Build history of the part. All positions in model axes, mm. A direction names the side the tool comes from. Give positions to 0.01 mm unless a question says otherwise; leave off trailing zeros. Loops run counter-clockwise (first coordinate to the right, second up) from the corner with the lowest first, then second, coordinate; pieces in that order, holes last. Notation, with made-up numbers: (41.25, -19) - (61.25, -19) arc R32 cw to (61.25, 13) - close; hole circle Ø5 at (21.25, 18). An arc over 180 degrees is marked (long way). Return JSON: item names as keys, results as strings. Group by question number.
1) Drill centre lines: probe 1 along X at (y, z) = (8, 28); probe 2 along Y at (x, z) = (-30.5, 8); probe 3 along Z at (x, y) = (-29, 7.75). Where is each one in solid material? Low to high. Write a range as from..to.
2) Slice it at B-B (z = 11). List the corners of the cut face in (x, y), and give its area (3 significant figures).
3) 3-axis set-ups, long thin cutter, end or side, ignore diameter. For faces 5 (the face through (-35, 15, 67)), 6 (the face through (0, 14, 35)): which of +Z, -Z, +X, -X, +Y, -Y reach the whole face in a straight line?
4) Drop flat-ended pins along their axis: pin 1 (8 mm diameter, centred on x = -42.5, y = 22, fed in from -Z); pin 2 (1.5 mm diameter, centred on x = -14.5, z = 21, fed in from -Y); pin 3 (6 mm diameter, centred on x = -13, z = 24.5, fed in from +Y); pin 4 (5 mm diameter, centred on x = -59, y = 21.5, fed in from -Z). Give the stop position or say it passes through.
5) Mould opens along Z. For faces 1 (the face through (-35, 0, 35)), 2 (the face through (-67, 15, 44)), 3 (the face through (-36.732, 14.11, 0.813)), 4 (the face through (-41.052, 14.035, -2.396)) say: released by +Z, released by -Z, zero draft, split by the parting line, or undercut.
6) Slice it at C-C (x = -24). List the corners of the cut face in (y, z).
7) Slice it at A-A (y = 5.75). List the corners of the cut face in (x, z).
```python
from build123d import *

# Parameters (mm, degrees)
BOSS_EXTRUDE1_DEPTH             = 3
BOSS_EXTRUDE2_DEPTH             = 25
SKETCH4_R                       = 2.5
BOSS_EXTRUDE3_DEPTH             = 7
BOSS_EXTRUDE3_DIRECTION_2_REACH = 85.256


with BuildPart() as part:
    # Sketch1 → Boss-Extrude1 (new body)
    with BuildSketch(Plane(origin=(0, 0, 0), x_dir=(1, 0, 0), z_dir=(0, 1, 0))):
        with BuildLine():
            Line((0, 0), (0, -70))
            Line((0, -70), (-70, -70))
            Line((-70, -70), (-70, -20))
            ThreePointArc((-70, -20), (-36.231761047, -5.688836334), (0, 0))
        make_face()
    extrude(amount=BOSS_EXTRUDE1_DEPTH)

    # Sketch2 → Boss-Extrude2 (add)
    with BuildSketch(Plane(origin=(0, 3, 0), x_dir=(1, 0, 0), z_dir=(0, 1, 0))):
        with BuildLine():
            Line((-70, -70), (0, -70))
            Line((0, -70), (0, 0))
            ThreePointArc((0, 0), (-36.231761047, -5.688836334), (-70, -20))
            Line((-70, -20), (-70, -70))
        make_face()
        with BuildLine():
            Line((-67, -21.744121307), (-67, -67))
            Line((-67, -67), (-3, -67))
            Line((-3, -67), (-3, -3.133993062))
            ThreePointArc((-3, -3.133993062), (-36.068657655, -8.763956776), (-67, -21.744121307))
        make_face(mode=Mode.SUBTRACT)
    extrude(amount=BOSS_EXTRUDE2_DEPTH)

    # Sketch4 → Boss-Extrude3 (add)
    with BuildSketch(Plane(origin=(-61.178699811, 14, 15.293872991), x_dir=(-0.8974903699241336, 0, 0.4410340529862088), z_dir=(-0.4410340529862088, 0, -0.8974903699241336))):
        with Locations((-25.829909239, 0)):
            Circle(SKETCH4_R)
    extrude(amount=BOSS_EXTRUDE3_DEPTH)

    # Sketch4 → Boss-Extrude3 direction 2 (add, up to next)
    with BuildSketch(Plane(origin=(-61.178699811, 14, 15.293872991), x_dir=(-0.8974903699241336, 0, 0.4410340529862088), z_dir=(-0.4410340529862088, 0, -0.8974903699241336)), mode=Mode.PRIVATE) as boss_extrude3_direction_2_sk1:
        with Locations((-25.829909239, 0)):
            Circle(SKETCH4_R)
    boss_extrude3_direction_2_tool1 = extrude(boss_extrude3_direction_2_sk1.sketch, amount=-BOSS_EXTRUDE3_DIRECTION_2_REACH, mode=Mode.PRIVATE) - part.part
    add(boss_extrude3_direction_2_tool1.solids().sort_by_distance((-37.996605, 14, 3.902003))[0])


solid = part.part
```
Results:
{
 "1": {"probe 1": "-70..-67, -3..0", "probe 2": "0..3", "probe 3": "3.82..6.9, 67..70"},
 "2": {"outline": "(-51.61, 0) - (0, 0) - (0, 28) - (-3, 28) - (-3, 3) - (-43.1, 3) - (-43.1, 28) - (-51.61, 28) - close", "area": "443 mm2"},
 "3": {"face 5": "+Y", "face 6": "+Z, -Z, +X, +Y, -Y"},
 "4": {"pin 1": "z = 6.36", "pin 2": "y = 0", "pin 3": "y = 3", "pin 4": "z = 13.09"},
 "5": {"face 1": "zero draft", "face 2": "undercut", "face 3": "undercut", "face 4": "released by -Z"},
 "6": {"outline": "(0, 2.74) - (28, 2.74) - (28, 5.8) - (3, 5.8) - (3, 67) - (28, 67) - (28, 70) - (0, 70) - close"},
 "7": {"outline": "(-70, 20) arc R150 ccw to (0, 0) - (0, 70) - (-70, 70) - close; hole (-67, 21.74) arc R147 ccw to (-3, 3.13) - (-3, 67) - (-67, 67) - close"}
}
